Build history of the part. All positions in model axes, mm. Give positions to 0.01 mm unless a question says otherwise; leave off trailing zeros. Loops run counter-clockwise (first coordinate to the right, second up) from the corner with the lowest first, then second, coordinate; pieces in that order, holes last. Notation, with made-up numbers: (-4, 21) -> (12, 21) arc R20 cw to (12, 36) -> close; hole circle Ø7 at (73.25, 70.5). An arc over 180 degrees is marked (long way). Answer as a JSON object with one key per item and string values. Group by question number.
from build123d import *

# Parameters (mm, degrees)
F1_DEPTH = 1


with BuildPart() as f1:
    # F0 (on Top) → F1 (new body)
    with BuildSketch(Plane.XY):
        with BuildLine():
            Line((-4.928222, -3.4827), (-3.4827, -4.928222))
            ThreePointArc((-3.4827, -4.928222), (-3.126054, -5.423345), (-3, -6.020383))
            Line((-3, -6.020383), (-3, -9.436451))
            ThreePointArc((-3, -9.436451), (0, -12.436451), (3, -9.436451))
            Line((3, -9.436451), (3, -6.020383))
            ThreePointArc((3, -6.020383), (3.126054, -5.423345), (3.4827, -4.928222))
            Line((3.4827, -4.928222), (4.928222, -3.4827))
            ThreePointArc((4.928222, -3.4827), (5.42923, -3.13937), (6.020383, -3))
            Line((6.020383, -3), (9.436451, -3))
            ThreePointArc((9.436451, -3), (12.436451, 0), (9.436451, 3))
            Line((9.436451, 3), (6.020383, 3))
            ThreePointArc((6.020383, 3), (5.42923, 3.13937), (4.928222, 3.4827))
            Line((4.928222, 3.4827), (3.4827, 4.928222))
            ThreePointArc((3.4827, 4.928222), (3.126054, 5.423345), (3, 6.020383))
            Line((3, 6.020383), (3, 9.436451))
            ThreePointArc((3, 9.436451), (0, 12.436451), (-3, 9.436451))
            Line((-3, 9.436451), (-3, 6.020383))
            ThreePointArc((-3, 6.020383), (-3.126054, 5.423345), (-3.4827, 4.928222))
            Line((-3.4827, 4.928222), (-4.928222, 3.4827))
            ThreePointArc((-4.928222, 3.4827), (-5.42923, 3.13937), (-6.020383, 3))
            Line((-6.020383, 3), (-9.436451, 3))
            ThreePointArc((-9.436451, 3), (-12.436451, 0), (-9.436451, -3))
            Line((-9.436451, -3), (-6.020383, -3))
            ThreePointArc((-6.020383, -3), (-5.42923, -3.13937), (-4.928222, -3.4827))
        make_face()
        with BuildLine():
            ThreePointArc((-1.500459, -7.936451), (0, -6.435991), (1.500459, -7.936451))
            Line((1.500459, -7.936451), (1.500459, -9.436451))
            ThreePointArc((1.500459, -9.436451), (0, -10.93691), (-1.500459, -9.436451))
            Line((-1.500459, -9.436451), (-1.500459, -7.936451))
        make_face(mode=Mode.SUBTRACT)
        with BuildLine():
            Line((-9.436451, 1.500459), (-7.936451, 1.500459))
            ThreePointArc((-7.936451, 1.500459), (-6.435991, 0), (-7.936451, -1.500459))
            Line((-7.936451, -1.500459), (-9.436451, -1.500459))
            ThreePointArc((-9.436451, -1.500459), (-10.93691, 0), (-9.436451, 1.500459))
        make_face(mode=Mode.SUBTRACT)
        with BuildLine():
            ThreePointArc((3.075914, 3.075914), (4.018876, 1.664673), (4.35, 0))
            ThreePointArc((4.35, 0), (-4.018876, -1.664673), (3.075914, 3.075914))
        make_face(mode=Mode.SUBTRACT)
        with BuildLine():
            Line((9.436451, -1.500459), (7.936451, -1.500459))
            ThreePointArc((7.936451, -1.500459), (6.435991, 0), (7.936451, 1.500459))
            Line((7.936451, 1.500459), (9.436451, 1.500459))
            ThreePointArc((9.436451, 1.500459), (10.93691, 0), (9.436451, -1.500459))
        make_face(mode=Mode.SUBTRACT)
        with BuildLine():
            Line((1.500459, 9.436451), (1.500459, 7.936451))
            ThreePointArc((1.500459, 7.936451), (0, 6.435991), (-1.500459, 7.936451))
            Line((-1.500459, 7.936451), (-1.500459, 9.436451))
            ThreePointArc((-1.500459, 9.436451), (0, 10.93691), (1.500459, 9.436451))
        make_face(mode=Mode.SUBTRACT)
    extrude(amount=F1_DEPTH)


solid = f1.part
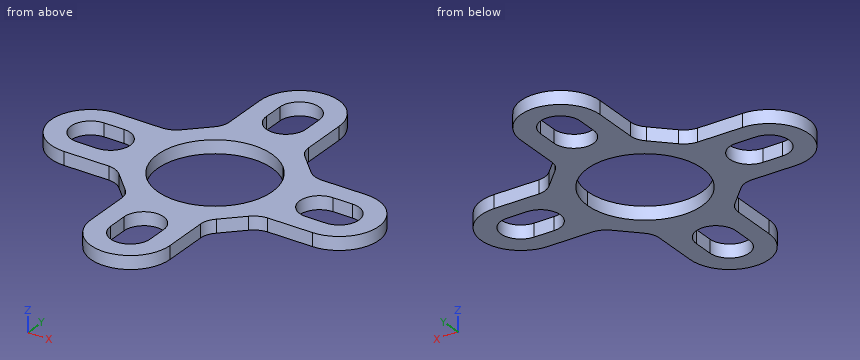
(1) Saw through at C-C on x = -7. List the corners of the cut face in (y, z), plus the area to 3 significant figures.
(2) Pin check, flat tips, straight feed: pin 1 (0.5 mm diameter, centred on x = -8.5, z = 0.5, fed in from +Y); pin 2 (0.5 mm diameter, centred on y = 7, z = 0.5, fed in from -X); pin 3 (0.5 mm diameter, centred on y = 8.5, z = 0.5, fed in from +X). Stop position of each tip, or through.
(3) Saw through at A-A on y = 7.5. List the corners of the cut face in (x, z).
(4) Saw through at B-B on x = 0. List the corners of the cut face in (y, z), plus the area to 3 significant figures.
(5) Saw through at D-D on z = 0.7. Give the number of separate pieces and of enclosed holes in the cut face, plus the area to 3 significant figures.
(6) Probe line 1 along X through (y, z) = (0, 0.25); line 2 along X through (y, z) = (-9, 0.6). List the from-to ranges inside material, lowest first. Write a range as [from, to].
Calculated:
{
 "1": {"outline": "(-3, 0) -> (-1.17, 0) -> (-1.17, 1) -> (-3, 1) -> close; (1.17, 0) -> (3, 0) -> (3, 1) -> (1.17, 1) -> close", "area": "3.66 mm^2"},
 "2": {"pin 1": "stops at y = 3", "pin 2": "stops at x = -3", "pin 3": "stops at x = 3"},
 "3": {"outline": "(-3, 0) -> (-1.44, 0) -> (-1.44, 1) -> (-3, 1) -> close; (1.44, 0) -> (3, 0) -> (3, 1) -> (1.44, 1) -> close"},
 "4": {"outline": "(-12.44, 0) -> (-10.94, 0) -> (-10.94, 1) -> (-12.44, 1) -> close; (-6.44, 0) -> (-4.35, 0) -> (-4.35, 1) -> (-6.44, 1) -> close; (4.35, 0) -> (6.44, 0) -> (6.44, 1) -> (4.35, 1) -> close; (10.94, 0) -> (12.44, 0) -> (12.44, 1) -> (10.94, 1) -> close", "area": "7.17 mm^2"},
 "5": {"separate pieces": "1", "enclosed holes": "5", "area": "153 mm^2"},
 "6": {"line 1": "x = [-12.44, -10.94], [-6.44, -4.35], [4.35, 6.44], [10.94, 12.44]", "line 2": "x = [-3, -1.5], [1.5, 3]"}
}
